from build123d import *

# Parameters (mm, degrees)
SKETCH1_R           = 10
SKETCH1_R_2         = 5
BOSS_EXTRUDE1_DEPTH = 10


with BuildPart() as part:
    # Sketch1 → Boss-Extrude1 (new body)
    with BuildSketch(Plane(origin=(0, 0, 0), x_dir=(-1, 0, 0), z_dir=(0, 1, 0))):
        with BuildLine():
            Line((8.4, -12.427389106), (49.824630354, 15.572610894))
            ThreePointArc((49.824630354, 15.572610894), (56.424630354, 28), (49.824630354, 40.427389106))
            Line((49.824630354, 40.427389106), (8.4, 68.427389106))
            ThreePointArc((8.4, 68.427389106), (-12.427389106, 64.4), (-8.4, 43.572610894))
            Line((-8.4, 43.572610894), (14.638916069, 28))
            Line((14.638916069, 28), (-8.4, 12.427389106))
            ThreePointArc((-8.4, 12.427389106), (-12.427389106, -8.4), (8.4, -12.427389106))
        make_face()
        with Locations(Location((0, 0, 0), (0, 0, 90))):
            Circle(SKETCH1_R, mode=Mode.SUBTRACT)
        with Locations(Location((0, 56, 0), (0, 0, 90))):
            Circle(SKETCH1_R_2, mode=Mode.SUBTRACT)
    extrude(amount=BOSS_EXTRUDE1_DEPTH)


solid = part.part
For this review, take the finished solid that the model builds, in its own axes (mm). A direction names the side the tool comes from. Round coordinates to 2 decimals unless told otherwise and drop trailing zeros. Write each loop counter-clockwise with the first axis right and the second up, starting at its lowest first coordinate (ties: lowest second). Pieces come first, ordered by that corner, then holes. Notation, with made-up numbers: (-37, -23.75) -> (17, -23.75) arc R22 ccw to (17, -12.75) -> close; hole circle Ø11 at (51, -21.75). An arc over 180 degrees is marked (long way). Put each result on its own line as item: value.
Q1. Consider section C-C on y = 7.25. State the section outline as (x, z) points.
Determined:
outline: (-49.82, 15.57) -> (-8.4, -12.43) arc R15 ccw to (8.4, 12.43) -> (-14.64, 28) -> (8.4, 43.57) arc R15 ccw to (-8.4, 68.43) -> (-49.82, 40.43) arc R15 ccw to start; hole circle Ø20 at (0, 0); hole circle Ø10 at (0, 56)
Q2. Machinability: for faces 5 (the flat face through (-2.958, 4.93, 35.895)), 6 (the flat face through (-29.402, 4.93, 54.231)), which of the approach directions +Z, -Z, +X, -X, +Y, -Y give a long, thin tool a straight path to every point of the face, cutting with its end or side? Answer none if there is none.
Determined:
face 5: +X, +Y, -Y
face 6: +Z, -X, +Y, -Y
Q3. Clearance check with flat-ended pins moving along their axes: pin 1 Ø2 at (x, y) = (-44.5, 2) entering from -Z; pin 2 Ø5 at (y, z) = (6.5, 58) entering from -X; pin 3 Ø6 at (x, y) = (-19, 8) entering from -Z. State where each tip first meets the part, or that it passes through.
Determined:
pin 1: stops at z = 11.3
pin 2: stops at x = -27.53
pin 3: stops at z = -7.29
Q4. The part is to be moulded in two halves that separate along Z. For faces 1 (the cylindrical face through (12, 5, 65)), 2 (the cylindrical face through (0, 5, 51)), 3 (the flat face through (-20, 10, 29)), 4 (the cylindrical face through (-56.423, 4.93, 27.795)), say which applies: released by +Z, released by -Z, zero draft, split by the parting line, or undercut.
Determined:
face 1: undercut
face 2: undercut
face 3: zero draft
face 4: split by the parting line
Q5. To check wall thickness, follow L1, parallel to Z at x = -4, y = 3; L2, parallel to Z at x = 8, y = 3.25; L3, parallel to Z at x = -6.5, y = 7.75. State the ranges of each line that lie inside material, in increasing order. Write a range as [from, to].
Determined:
L1: z = [-14.46, -9.17], [9.17, 20.81], [35.19, 53], [59, 70.46]
L2: z = [-12.69, -6], [6, 12.7], [43.3, 68.69]
L3: z = [-13.52, -7.6], [7.6, 22.5], [33.5, 69.52]
Q6. Consider section B-B on z = 52.5. State the section outline as (x, y) points, and give its area (3 significant figures).
Determined:
outline: (-31.96, 0) -> (-3.57, 0) -> (-3.57, 10) -> (-31.96, 10) -> close; (3.57, 0) -> (14.59, 0) -> (14.59, 10) -> (3.57, 10) -> close
area: 394 mm^2
Q7. Consider section D-D on z = 0. State the section outline as (x, y) points, and give its area (3 significant figures).
Determined:
outline: (-26.79, 0) -> (-10, 0) -> (-10, 10) -> (-26.79, 10) -> close; (10, 0) -> (15, 0) -> (15, 10) -> (10, 10) -> close
area: 218 mm^2
Q8. Consider section A-A on x = 0. State the section outline as (y, z) points, and give its area (3 significant figures).
Determined:
outline: (0, -15) -> (10, -15) -> (10, -10) -> (0, -10) -> close; (0, 10) -> (10, 10) -> (10, 18.11) -> (0, 18.11) -> close; (0, 37.89) -> (10, 37.89) -> (10, 51) -> (0, 51) -> close; (0, 61) -> (10, 61) -> (10, 71) -> (0, 71) -> close
area: 362 mm^2
